Verification items for the finished model (mm, model axes). Face numbers are marked on the shaded views. Give positions to 0.01 mm unless a question says otherwise; leave off trailing zeros. Order: outer loops, then holes, each group sorted by start corner. A loop starts at its lowest first (then second) coordinate and runs counter-clockwise, first axis right, second up.
(1) Sectioned sample at C-C on x = 57.5. Record the cut outline in (y, z).
(2) Mould release check, pull along Z, two halves, no side actions. Record for the marked faces 1, 2 and 3: pulls with the +Z half, pulls with the -Z half, needs draft (parallel to the pull), parting line crosses it, or undercut.
(3) Sectioned sample at A-A on y = 8.5. Count the separate pieces of the cut face and the enclosed holes in it, plus the area to 3 significant figures.
(4) Scan lines: L1, parallel to X at y = 4.75, z = -44; L2, parallel to Z at x = 27, y = 9; L3, parallel to X at y = 8.5, z = -51. Record each from-to range of solid material in increasing order.
(5) Sectioned sample at B-B on z = -43. Record the cut outline in (x, y).
(6) Sectioned sample at D-D on z = -55. Record the cut outline in (x, y), plus the area to 3 significant figures.
(7) Gauge pin test, flat end, axial feed: pin 1 (1.9 mm diameter, centred on x = 40, y = 16, fed in from +Z). Record the tip position at first contact, or that the pin passes through.
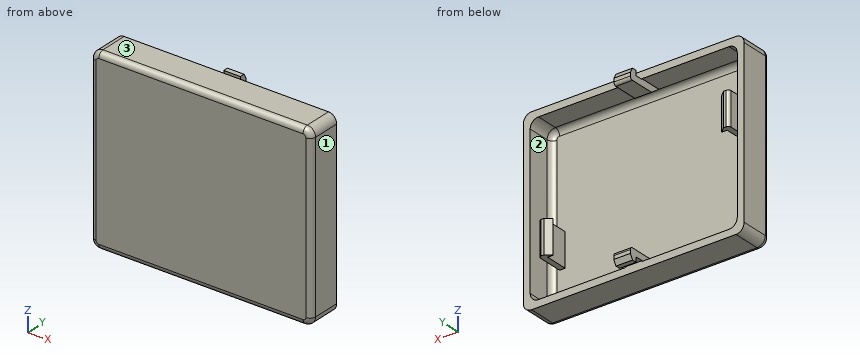
```python
from build123d import *

# Parameters (mm, degrees)
SKETCH1_W            = 80
SKETCH1_H            = 65
BOSS_EXTRUDE1_DEPTH  = 12
SKETCH2_W            = 75
SKETCH2_H            = 60
CUT_EXTRUDE1_DEPTH   = 10
FILLET4_R            = 2
FILLET5_R            = 3
FILLET8_R            = 2
SKETCH5_W            = 6
SKETCH5_H            = 13.5
BOSS_EXTRUDE2_DEPTH  = 2.5
CUT_EXTRUDE3_REACH   = 81.876
SKETCH6_W            = 0.25
SKETCH6_H            = 5.5
BOSS_EXTRUDE3_DEPTH  = 6
CUT_EXTRUDE4_REACH   = 81.876
SKETCH10_W           = 6
SKETCH10_H           = 13.5
BOSS_EXTRUDE4_DEPTH  = 2.5
CUT_EXTRUDE5_REACH   = 81.876
SKETCH11_W           = 0.25
SKETCH11_H           = 5.5
BOSS_EXTRUDE5_DEPTH  = 6
CUT_EXTRUDE6_DEPTH   = 6
SKETCH14_W           = 2
SKETCH14_H           = 12
BOSS_EXTRUDE7_DEPTH  = 10
SKETCH15_W           = 12
SKETCH15_H           = 1.75
BOSS_EXTRUDE8_DEPTH  = 2
SKETCH16_W           = 2
SKETCH16_H           = 12
BOSS_EXTRUDE9_DEPTH  = 10
SKETCH17_W           = 12
SKETCH17_H           = 1.75
BOSS_EXTRUDE10_DEPTH = 2
FILLET9_R            = 1
CUT_EXTRUDE7_REACH   = 97.176
CUT_EXTRUDE8_REACH   = 91.658


with BuildPart() as part:
    # Sketch1 → Boss-Extrude1 (new body)
    with BuildSketch(Plane(origin=(0, 0, 0), x_dir=(1, 0, 0), z_dir=(0, 1, 0))):
        with Locations((40, 32.5)):
            Rectangle(SKETCH1_W, SKETCH1_H)
    extrude(amount=BOSS_EXTRUDE1_DEPTH)

    # Sketch2 → Cut-Extrude1 (cut)
    with BuildSketch(Plane(origin=(0, 12, 0), x_dir=(1, 0, 0), z_dir=(0, 1, 0))):
        with Locations((40, 32.5)):
            Rectangle(SKETCH2_W, SKETCH2_H)
    extrude(amount=-CUT_EXTRUDE1_DEPTH, mode=Mode.SUBTRACT)

    # Fillet4
    fillet4_edges = [part.edges().sort_by_distance(p)[0] for p in [
        (40, 0, -65),
        (80, 0, -32.5),
        (40, 0, 0),
        (0, 0, -32.5),
    ]]
    fillet(fillet4_edges, radius=FILLET4_R)

    # Fillet5
    # the kernel refuses this fillet: 3 mm, written as the material it adds along each edge
    with BuildSketch(Plane(origin=(2.5, 12, -2.5), x_dir=(0, 0, -1), z_dir=(0, -1, 0)), Plane(origin=(77.5, 12, -62.5), x_dir=(0, 0, 1), z_dir=(0, -1, 0)), Plane(origin=(77.5, 12, -2.5), x_dir=(-1, 0, 0), z_dir=(0, -1, 0))) as fillet5_piece_1:
        with BuildLine():
            CenterArc((FILLET5_R, FILLET5_R), FILLET5_R, 180, 90)
            Line((0, FILLET5_R), (0, 0))
            Line((0, 0), (FILLET5_R, 0))
        make_face()
    extrude(amount=10)
    with BuildSketch(Plane(origin=(2.5, 12, -62.5), x_dir=(0, 0, 1), z_dir=(0, -1, 0))) as fillet5_piece_2:
        with BuildLine():
            CenterArc((FILLET5_R, -FILLET5_R), FILLET5_R, 90, 90)
            Line((0, -FILLET5_R), (0, 0))
            Line((0, 0), (FILLET5_R, 0))
        make_face()
    extrude(amount=10)
    # the kernel refuses this fillet: 3 mm, written as the material it takes off along each edge
    with BuildSketch(Plane(origin=(77, 0, -62), x_dir=(0, 0, -1), z_dir=(-1, 0, 0))) as fillet5_2_piece_1:
        with BuildLine():
            CenterArc((1, -2), 2, 0, 90)
            Line((3, -2), (3, 0))
            Line((3, 0), (1, 0))
        make_face()
    revolve(axis=Axis((77, 0, -62), (0, -1, 0)), revolution_arc=90, mode=Mode.SUBTRACT)
    with BuildSketch(Plane(origin=(77, 0, -3), x_dir=(1, 0, 0), z_dir=(0, 0, -1))) as fillet5_2_piece_2:
        with BuildLine():
            CenterArc((1, -2), 2, 0, 90)
            Line((3, -2), (3, 0))
            Line((3, 0), (1, 0))
        make_face()
    revolve(axis=Axis((77, 0, -3), (0, -1, 0)), revolution_arc=90, mode=Mode.SUBTRACT)
    with BuildSketch(Plane(origin=(3, 0, -62), x_dir=(-1, 0, 0), z_dir=(0, 0, 1))) as fillet5_2_piece_3:
        with BuildLine():
            CenterArc((1, -2), 2, 0, 90)
            Line((3, -2), (3, 0))
            Line((3, 0), (1, 0))
        make_face()
    revolve(axis=Axis((3, 0, -62), (0, -1, 0)), revolution_arc=90, mode=Mode.SUBTRACT)
    with BuildSketch(Plane(origin=(3, 0, -3), x_dir=(0, 0, 1), z_dir=(1, 0, 0))) as fillet5_2_piece_4:
        with BuildLine():
            CenterArc((1, -2), 2, 0, 90)
            Line((3, -2), (3, 0))
            Line((3, 0), (1, 0))
        make_face()
    revolve(axis=Axis((3, 0, -3), (0, -1, 0)), revolution_arc=90, mode=Mode.SUBTRACT)
    with BuildSketch(Plane(origin=(0, 0, -65), x_dir=(0, 0, 1), z_dir=(0, 1, 0)), Plane(origin=(0, 0, 0), x_dir=(1, 0, 0), z_dir=(0, 1, 0))) as fillet5_2_piece_5:
        with BuildLine():
            CenterArc((FILLET5_R, FILLET5_R), FILLET5_R, 180, 90)
            Line((0, FILLET5_R), (0, 0))
            Line((0, 0), (FILLET5_R, 0))
        make_face()
    extrude(amount=19.5, mode=Mode.SUBTRACT)
    with BuildSketch(Plane(origin=(80, 0, -65), x_dir=(0, 0, 1), z_dir=(0, 1, 0)), Plane(origin=(80, 0, 0), x_dir=(-1, 0, 0), z_dir=(0, 1, 0))) as fillet5_2_piece_6:
        with BuildLine():
            CenterArc((FILLET5_R, -FILLET5_R), FILLET5_R, 90, 90)
            Line((0, -FILLET5_R), (0, 0))
            Line((0, 0), (FILLET5_R, 0))
        make_face()
    extrude(amount=19.5, mode=Mode.SUBTRACT)

    # Fillet8
    fillet8_edges = [part.edges().sort_by_distance(p)[0] for p in [
        (40, 2, -2.5),
        (2.5, 2, -32.5),
        (77.5, 2, -32.5),
        (40, 2, -62.5),
        (3.378679656, 2, -61.621320344),
        (76.621320344, 2, -61.621320344),
        (76.621320344, 2, -3.378679656),
        (3.378679656, 2, -3.378679656),
    ]]
    fillet(fillet8_edges, radius=FILLET8_R)

    # Sketch5 → Boss-Extrude2 (add)
    with BuildSketch(Plane.XY.offset(-62.5)):
        with Locations((40, 10.75)):
            Rectangle(SKETCH5_W, SKETCH5_H)
    extrude(amount=BOSS_EXTRUDE2_DEPTH)

    # Sketch6 → Cut-Extrude3 (cut, up to next)
    with BuildSketch(Plane(origin=(43, 0, 0), x_dir=(0, 0, -1), z_dir=(1, 0, 0)), mode=Mode.PRIVATE) as cut_extrude3_sk1:
        with Locations((62.375, 14.75)):
            Rectangle(SKETCH6_W, SKETCH6_H)
    cut_extrude3_tool1 = extrude(cut_extrude3_sk1.sketch, amount=-CUT_EXTRUDE3_REACH, mode=Mode.PRIVATE) & part.part
    add(cut_extrude3_tool1.solids().sort_by_distance((43, 14.75, -62.375))[0], mode=Mode.SUBTRACT)

    # Sketch7 → Boss-Extrude3 (add)
    with BuildSketch(Plane(origin=(43, 0, 0), x_dir=(0, 0, -1), z_dir=(1, 0, 0))):
        Polygon((62.25, 14.75), (64, 14.75), (64, 16.5), (62.25, 17.5), align=None)
    extrude(amount=-BOSS_EXTRUDE3_DEPTH)

    # Sketch8 → Cut-Extrude4 (cut, up to next)
    with BuildSketch(Plane(origin=(43, 0, 0), x_dir=(0, 0, -1), z_dir=(1, 0, 0)), mode=Mode.PRIVATE) as cut_extrude4_sk1:
        Polygon((60, 4), (62.5, 4), (60, 7.5), align=None)
    cut_extrude4_tool1 = extrude(cut_extrude4_sk1.sketch, amount=-CUT_EXTRUDE4_REACH, mode=Mode.PRIVATE) & part.part
    add(cut_extrude4_tool1.solids().sort_by_distance((43, 5.166667, -60.833333))[0], mode=Mode.SUBTRACT)

    # Sketch10 → Boss-Extrude4 (add)
    with BuildSketch(Plane(origin=(0, 0, -2.5), x_dir=(-1, 0, 0), z_dir=(0, 0, -1))):
        with Locations((-40, 10.75)):
            Rectangle(SKETCH10_W, SKETCH10_H)
    extrude(amount=BOSS_EXTRUDE4_DEPTH)

    # Sketch11 → Cut-Extrude5 (cut, up to next)
    with BuildSketch(Plane.ZY.offset(-37), mode=Mode.PRIVATE) as cut_extrude5_sk1:
        with Locations((-2.625, 14.75)):
            Rectangle(SKETCH11_W, SKETCH11_H)
    cut_extrude5_tool1 = extrude(cut_extrude5_sk1.sketch, amount=-CUT_EXTRUDE5_REACH, mode=Mode.PRIVATE) & part.part
    add(cut_extrude5_tool1.solids().sort_by_distance((37, 14.75, -2.625))[0], mode=Mode.SUBTRACT)

    # Sketch12 → Boss-Extrude5 (add)
    with BuildSketch(Plane.ZY.offset(-37)):
        Polygon((-2.75, 14.75), (-1, 14.75), (-1, 16.5), (-2.75, 17.5), align=None)
    extrude(amount=-BOSS_EXTRUDE5_DEPTH)

    # Sketch13 → Cut-Extrude6 (cut)
    with BuildSketch(Plane.ZY.offset(-37)):
        Polygon((-5, 4), (-2.5, 4), (-5, 7.5), align=None)
    extrude(amount=-CUT_EXTRUDE6_DEPTH, mode=Mode.SUBTRACT)

    # Sketch14 → Boss-Extrude7 (add)
    with BuildSketch(Plane(origin=(0, 2, 0), x_dir=(1, 0, 0), z_dir=(0, 1, 0))):
        with Locations((6.5, 22.5)):
            Rectangle(SKETCH14_W, SKETCH14_H)
    extrude(amount=BOSS_EXTRUDE7_DEPTH)

    # Sketch15 → Boss-Extrude8 (add)
    with BuildSketch(Plane(origin=(7.5, 0, 0), x_dir=(0, 0, -1), z_dir=(1, 0, 0))):
        with Locations((22.5, 11.125)):
            Rectangle(SKETCH15_W, SKETCH15_H)
    extrude(amount=BOSS_EXTRUDE8_DEPTH)

    # Sketch16 → Boss-Extrude9 (add)
    with BuildSketch(Plane(origin=(0, 2, 0), x_dir=(1, 0, 0), z_dir=(0, 1, 0))):
        with Locations((73.5, 42.5)):
            Rectangle(SKETCH16_W, SKETCH16_H)
    extrude(amount=BOSS_EXTRUDE9_DEPTH)

    # Sketch17 → Boss-Extrude10 (add)
    with BuildSketch(Plane.ZY.offset(-72.5)):
        with Locations((-42.5, 11.125)):
            Rectangle(SKETCH17_W, SKETCH17_H)
    extrude(amount=BOSS_EXTRUDE10_DEPTH)

    # Fillet9
    fillet9_edges = [part.edges().sort_by_distance(p)[0] for p in [
        (40, 17.5, -60),
        (40, 17.5, -5),
        (5.5, 12, -22.5),
        (74.5, 12, -42.5),
    ]]
    fillet(fillet9_edges, radius=FILLET9_R)

    # Sketch18 → Cut-Extrude7 (cut, up to next)
    with BuildSketch(Plane.XY.offset(-16.5), mode=Mode.PRIVATE) as cut_extrude7_sk1:
        Polygon((7.5, 12), (9.5, 10.25), (9.5, 12), align=None)
    cut_extrude7_tool1 = extrude(cut_extrude7_sk1.sketch, amount=-CUT_EXTRUDE7_REACH, mode=Mode.PRIVATE) & part.part
    add(cut_extrude7_tool1.solids().sort_by_distance((8.833333, 11.416667, -16.5))[0], mode=Mode.SUBTRACT)

    # Sketch19 → Cut-Extrude8 (cut, up to next)
    with BuildSketch(Plane.XY.offset(-36.5), mode=Mode.PRIVATE) as cut_extrude8_sk1:
        Polygon((70.5, 10.25), (72.5, 12), (70.5, 12), align=None)
    cut_extrude8_tool1 = extrude(cut_extrude8_sk1.sketch, amount=-CUT_EXTRUDE8_REACH, mode=Mode.PRIVATE) & part.part
    add(cut_extrude8_tool1.solids().sort_by_distance((71.166667, 11.416667, -36.5))[0], mode=Mode.SUBTRACT)


solid = part.part
```
Ans:
1. outline: (0, -63) arc R2 ccw to (2, -65) - (12, -65) - (12, -62.5) - (4, -62.5) arc R2 cw to (2, -60.5) - (2, -4.5) arc R2 cw to (4, -2.5) - (12, -2.5) - (12, 0) - (2, 0) arc R2 ccw to (0, -2) - close
2. face 1: needs draft
2. face 2: undercut
2. face 3: pulls with the +Z half
3. separate pieces: 3
3. enclosed holes: 1
3. area: 778 mm2
4. L1: x = 0 to 2.5, 72.5 to 74.5, 77.5 to 80
4. L2: z = -65 to -62.5, -2.5 to 0
4. L3: x = 0 to 2.5, 77.5 to 80
5. outline: (0, 2) arc R2 ccw to (2, 0) - (78, 0) arc R2 ccw to (80, 2) - (80, 12) - (77.5, 12) - (77.5, 4) arc R2 cw to (75.5, 2) - (74.5, 2) - (74.5, 11) arc R1 ccw to (73.5, 12) - (72.5, 12) - (70.5, 10.25) - (72.5, 10.25) - (72.5, 2) - (4.5, 2) arc R2 cw to (2.5, 4) - (2.5, 12) - (0, 12) - close
6. outline: (0, 2) arc R2 ccw to (2, 0) - (78, 0) arc R2 ccw to (80, 2) - (80, 12) - (77.5, 12) - (77.5, 4) arc R2 cw to (75.5, 2) - (4.5, 2) arc R2 cw to (2.5, 4) - (2.5, 12) - (0, 12) - close
6. area: 210 mm2
7. pin 1: stops at z = -1
